from build123d import *

# Parameters (mm, degrees)
CYLINDER003_R     = 1.65
CYLINDER003_DEPTH = 2.55
BOX004_W          = 33
BOX004_H          = 2.55
BOX004_DEPTH      = 7


with BuildPart() as hole001:
    # Cylinder003 → Cylinder003 (new body)
    with BuildSketch(Plane(origin=(3.5, -22.5, 9), x_dir=(1, 0, 0), z_dir=(0, 0, 1))):
        Circle(CYLINDER003_R)
    extrude(amount=CYLINDER003_DEPTH)


with BuildPart() as hole005:
    # Clone012 base: copy of hole001
    add(hole001.part)


with BuildPart() as hole005_1:
    # Clone012 placement: moved
    add(hole005.part.moved(Location((26, 0, 0))))


with BuildPart() as fusion002:
    # Fusion002 base: copy of hole001
    add(hole001.part)

    # Fusion002: union hole005
    add(hole005_1.part)


with BuildPart() as obj1:
    # Box004 → Box004 (new body)
    with BuildSketch(Plane(origin=(0, -19, 9), x_dir=(1, 0, 0), z_dir=(0, -1, 0))):
        with Locations((16.5, 1.275)):
            Rectangle(BOX004_W, BOX004_H)
    extrude(amount=BOX004_DEPTH)

    # Cut002: cut Fusion002
    add(fusion002.part, mode=Mode.SUBTRACT)


solid = obj1.part
The model under review builds one solid part; all positions refer to its coordinate system, in mm. Give positions to 0.01 mm unless a question says otherwise; leave off trailing zeros. Write each loop counter-clockwise with the first axis right and the second up, starting at its lowest first coordinate (ties: lowest second). Pieces come first, ordered by that corner, then holes.
1. Add section B-B, the plane y = -22.5. Write out the cut boundary in (x, z), plus the area to 3 significant figures.
2. For P1, Ø1, axis at y = -20.5, z = 10.5, coming from the -X side; P2, Ø3, axis at x = 29.5, y = -22.5, coming from the -Z side, all flat-tipped, find the tip position at first contact; note any pin that passes through.
3. Add section C-C, the plane z = 10.65. Write out the cut boundary in (x, y), plus the area to 3 significant figures.
4. Draft analysis for pull direction X (two halves, no side actions). For faces 1 (the flat face through (0, -22, 10)), 2 (the flat face through (16, -26, 10)), 3 (the cylindrical face through (28.284, -21.385, 10.257)), state which applies: +X half, -X half, draft (parallel to the pull), parting line (faces both ways), or undercut.
5. Wall thickness on L1, parallel to Y at x = 3.5, z = 10.1; L2, parallel to X at y = -24, z = 9.6; L3, parallel to X at y = -22.25, z = 10.6: over which ranges is each line inside the solid? List them lowest first.
6. Add section A-A, the plane x = 29.5. Write out the cut boundary in (y, z).
7. Add section D-D, the plane y = -23.75. Write out the cut boundary in (x, z).
Worked answers:
1. outline: (0, 9) - (1.85, 9) - (1.85, 11.55) - (0, 11.55) - close; (5.15, 9) - (27.85, 9) - (27.85, 11.55) - (5.15, 11.55) - close; (31.15, 9) - (33, 9) - (33, 11.55) - (31.15, 11.55) - close
1. area: 67.3 mm2
2. P1: stops at x = 0
2. P2: passes through
3. outline: (0, -26) - (33, -26) - (33, -19) - (0, -19) - close; hole circle Ø3.3 at (3.5, -22.5); hole circle Ø3.3 at (29.5, -22.5)
3. area: 214 mm2
4. face 1: -X half
4. face 2: draft
4. face 3: undercut
5. L1: y = -26 to -24.15, -20.85 to -19
5. L2: x = 0 to 2.81, 4.19 to 28.81, 30.19 to 33
5. L3: x = 0 to 1.87, 5.13 to 27.87, 31.13 to 33
6. outline: (-26, 9) - (-24.15, 9) - (-24.15, 11.55) - (-26, 11.55) - close; (-20.85, 9) - (-19, 9) - (-19, 11.55) - (-20.85, 11.55) - close
7. outline: (0, 9) - (2.42, 9) - (2.42, 11.55) - (0, 11.55) - close; (4.58, 9) - (28.42, 9) - (28.42, 11.55) - (4.58, 11.55) - close; (30.58, 9) - (33, 9) - (33, 11.55) - (30.58, 11.55) - close
